Geometry: final body of the model. Coordinates: model frame, mm. A direction names the side the tool comes from. Give positions to 0.01 mm unless a question says otherwise; leave off trailing zeros. Order: outer loops, then holes, each group sorted by start corner. A loop starts at its lowest first (then second) coordinate and runs counter-clockwise, first axis right, second up. Notation, with made-up numbers: M 26,63.5 L 83,63.5 A19 ccw 83,80.5 Z; hole C 23,49.25 d11. An arc over 180 degrees is marked long. One line per item, written item: value. Start each with the question number.
```python
from build123d import *

# Parameters (mm, degrees)
SKETCH_1_W          = 46
SKETCH_1_H          = 20
SKETCH_1_R          = 1.6
EXTRUDE_1_DEPTH     = 1.5
SKETCH_2_W          = 29.5
SKETCH_2_H          = 10
CUT_EXTRUDE_1_DEPTH = 0.25
SKETCH_3_W          = 11.5
SKETCH_3_H          = 8
CUT_EXTRUDE_2_DEPTH = 30.25


with BuildPart() as part:
    # 草图1 → 凸台-拉伸1 (new body)
    with BuildSketch(Plane(origin=(0, 0, 0), x_dir=(1, 0, 0), z_dir=(0, 1, 0))):
        Rectangle(SKETCH_1_W, SKETCH_1_H)
        with Locations(Location((-19.5, 7, 0), (0, 0, 270))):
            Circle(SKETCH_1_R, mode=Mode.SUBTRACT)
        with Locations(Location((19.5, 7, 0), (0, 0, 90))):
            Circle(SKETCH_1_R, mode=Mode.SUBTRACT)
        with Locations(Location((19.5, -7, 0), (0, 0, 270))):
            Circle(SKETCH_1_R, mode=Mode.SUBTRACT)
        with Locations(Location((-19.5, -7, 0), (0, 0, 90))):
            Circle(SKETCH_1_R, mode=Mode.SUBTRACT)
    extrude(amount=EXTRUDE_1_DEPTH)

    # 草图2 → 切除-拉伸1 (cut)
    with BuildSketch(Plane(origin=(0, 1.5, 0), x_dir=(1, 0, 0), z_dir=(0, 1, 0))):
        with Locations((8.25, 0)):
            Rectangle(SKETCH_2_W, SKETCH_2_H)
    extrude(amount=-CUT_EXTRUDE_1_DEPTH, mode=Mode.SUBTRACT)

    # 草图3 → 切除-拉伸2 (cut)
    with BuildSketch(Plane(origin=(0, 1.25, 0), x_dir=(1, 0, 0), z_dir=(0, 1, 0))):
        with Locations((17.25, 0)):
            Rectangle(SKETCH_3_W, SKETCH_3_H)
    extrude(amount=-CUT_EXTRUDE_2_DEPTH, mode=Mode.SUBTRACT)


solid = part.part
```
Q1. Set-up query: faces 5 (the face through (-23, 1, 0)), 6 (the face through (17, 1, 4)), 7 (the face through (5, 1.25, 0)). Return all of +Z, -Z, +X, -X, +Y, -Y with unobstructed straight access to the full face (end or side cutting, diameter ignored); none if empty.
Q2. Ray query, line 1 along X through (y, z) = (0.95, 7); line 2 along X through (y, z) = (1.05, -6); line 3 along Z through (x, y) = (13.5, 0.3). Return the intervals inside material, ascending. Write a range as [from, to].
Q3. Section query D-D on x = -19.5. Return loops of the section in (y, z), and give its area (3 significant figures).
Q4. Section query A-A on x = 19.5. Return loops of the section in (y, z).
Q5. Mould query, pull axis Z, two halves, no side actions, for faces 1 (the face through (11.5, 1, 0)), 2 (the face through (23, 1, -7)), 3 (the face through (0, 1, -10)), 4 (the face through (-17.914, 0.74, -7.208)). Classes: +Z half, -Z half, draft (parallel to the pull), parting line (faces both ways), or undercut.
Q6. Section query B-B on z = 7. Return loops of the section in (x, y).
Q7. Section query C-C on y = 0.85. Return loops of the section in (x, z).
Q8. Contact query for a flat-ended pin moving along its axis: pin 1 (1.9 mm diameter, centred on x = -19.5, z = -7, fed in from +Y). Output: stop coordinate, or through.
Results below:
1. face 5: +Z, -Z, -X, +Y, -Y
1. face 6: +X, +Y, -Y
1. face 7: +X, +Y
2. line 1: [-23, -21.1], [-17.9, 17.9], [21.1, 23]
2. line 2: [-23, -20.75], [-18.25, 18.25], [20.75, 23]
2. line 3: [-10, -4], [4, 10]
3. outline: M 0,-10 L 1.5,-10 L 1.5,-8.6 L 0,-8.6 Z; M 0,-5.4 L 1.5,-5.4 L 1.5,5.4 L 0,5.4 Z; M 0,8.6 L 1.5,8.6 L 1.5,10 L 0,10 Z
3. area: 20.4 mm2
4. outline: M 0,-10 L 1.5,-10 L 1.5,-8.6 L 0,-8.6 Z; M 0,-5.4 L 1.5,-5.4 L 1.5,-5 L 1.25,-5 L 1.25,-4 L 0,-4 Z; M 0,4 L 1.25,4 L 1.25,5 L 1.5,5 L 1.5,5.4 L 0,5.4 Z; M 0,8.6 L 1.5,8.6 L 1.5,10 L 0,10 Z
5. face 1: undercut
5. face 2: draft
5. face 3: -Z half
5. face 4: undercut
6. outline: M -23,0 L -21.1,0 L -21.1,1.5 L -23,1.5 Z; M -17.9,0 L 17.9,0 L 17.9,1.5 L -17.9,1.5 Z; M 21.1,0 L 23,0 L 23,1.5 L 21.1,1.5 Z
7. outline: M -23,-10 L 23,-10 L 23,-4 L 11.5,-4 L 11.5,4 L 23,4 L 23,10 L -23,10 Z; hole C -19.5,-7 d3.2; hole C -19.5,7 d3.2; hole C 19.5,-7 d3.2; hole C 19.5,7 d3.2
8. pin 1: through
